Print and shaded views of the part. All mm, measured from the part's lowest x, y and z. Round coordinates to 2 decimals unless told otherwise and drop trailing zeros. Write each loop counter-clockwise with the first axis right and the second up, starting at its lowest first coordinate (ties: lowest second). Pieces come first, ordered by that corner, then holes.
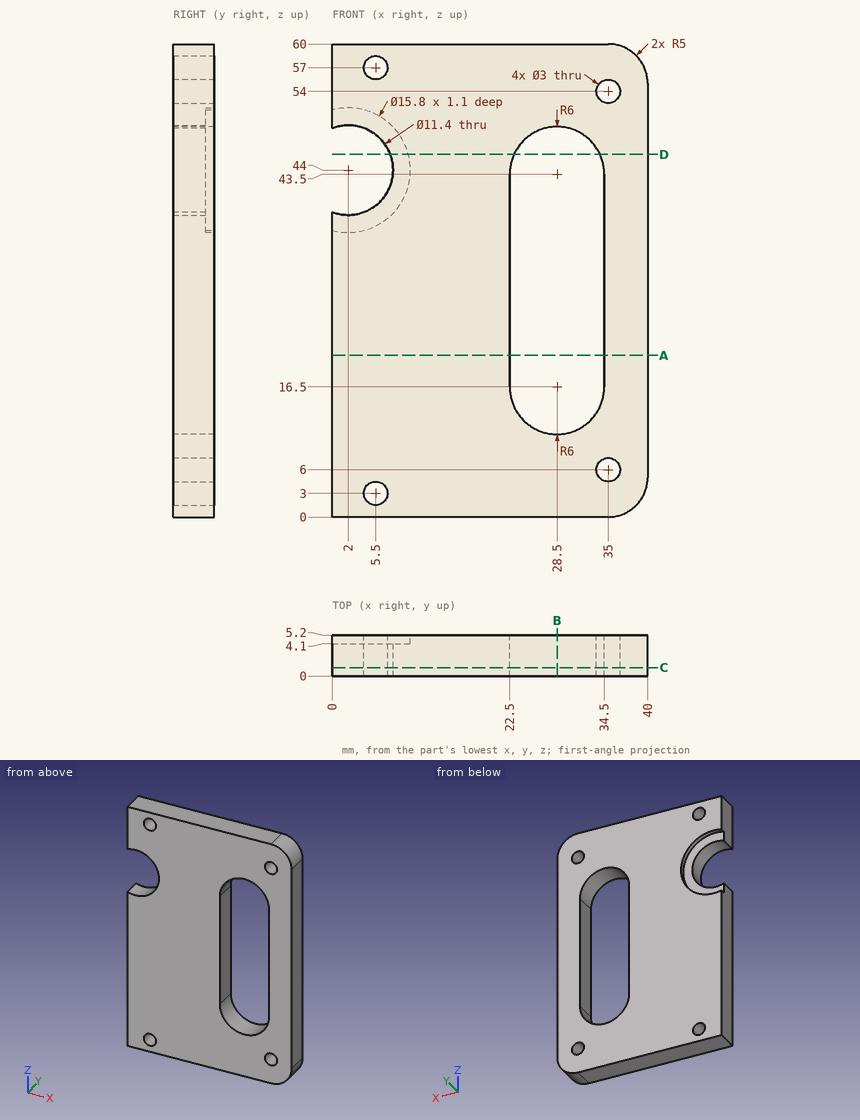
1) Slice it at A-A (z = 20.5). Write the cut outline in (x, y).
Results:
outline: (0, 0) - (22.5, 0) - (22.5, 5.2) - (0, 5.2) - close; (34.5, 0) - (40, 0) - (40, 5.2) - (34.5, 5.2) - close
2) Pin check, flat tips, straight feed: pin 1 Ø3 at (x, z) = (5.5, 44) entering from +Y; pin 2 Ø4 at (x, z) = (5.5, 3) entering from +Y. Stop position of each tip, or through.
Results:
pin 1: passes through
pin 2: stops at y = 5.2
3) Wall check: L1, parallel to X at y = 4.5, z = 35; L2, parallel to X at y = 2.95, z = 54; L3, parallel to Z at x = 5, y = 3.85. Give the ranges that are in metal, low to high.
Results:
L1: x = 0 to 22.5, 34.5 to 40
L2: x = 0 to 33.5, 36.5 to 40
L3: z = 0 to 1.59, 4.41 to 39.15, 48.85 to 55.59, 58.41 to 60
4) Slice it at C-C (y = 1.05). Write the cut outline in (x, z), plus the area to 3 significant figures.
Results:
outline: (0, 0) - (35, 0) arc R5 ccw to (40, 5) - (40, 55) arc R5 ccw to (35, 60) - (0, 60) - (0, 49.34) arc R5.7 cw (long way) to (0, 38.66) - close; hole circle Ø3 at (5.5, 3); hole circle Ø3 at (5.5, 57); hole (22.5, 16.5) arc R6 ccw to (34.5, 16.5) - (34.5, 43.5) arc R6 ccw to (22.5, 43.5) - close; hole circle Ø3 at (35, 6); hole circle Ø3 at (35, 54)
area: 1,850 mm2
5) Slice it at D-D (z = 46). Write the cut outline in (x, y).
Results:
outline: (7.34, 0) - (23.05, 0) - (23.05, 5.2) - (9.64, 5.2) - (9.64, 4.1) - (7.34, 4.1) - close; (33.95, 0) - (40, 0) - (40, 5.2) - (33.95, 5.2) - close
6) Slice it at B-B (x = 28.5). Write the cut outline in (y, z), plus the area to 3 significant figures.
Results:
outline: (0, 0) - (5.2, 0) - (5.2, 10.5) - (0, 10.5) - close; (0, 49.5) - (5.2, 49.5) - (5.2, 60) - (0, 60) - close
area: 109 mm2
